from build123d import *

# Parameters (mm, degrees)
KES_EKSTR_ZYON1_DEPTH      = 49.846698967
KES_EKSTR_ZYON1_DEPTH_BACK = 49.846698967
PAH1_SIZE                  = 1


with BuildPart() as part:
    # Çizim1 → Döndür1 (revolve)
    with BuildSketch(Plane.XY, mode=Mode.PRIVATE) as d_nd_r1_sk:
        Polygon((0, 0), (0, 15), (-6, 15), (-6, 11), (-19, 11), (-19, 9), (-22, 9), (-22, 10), (-44, 10), (-44, 0), align=None)
    revolve(d_nd_r1_sk.sketch.rotate(Axis((0, 0, 0), (-1, 0, 0)), 90), axis=Axis((0, 0, 0), (-1, 0, 0)))

    # Çizim2 → Kes-Ekstrüzyon1 (cut, two sides: drawn at the far end of the back side and taken through both)
    with BuildSketch(Plane(origin=(0, 0, 0), x_dir=(1, 0, 0), z_dir=(0, 1, 0)).offset(-KES_EKSTR_ZYON1_DEPTH_BACK)):
        Polygon((0, 0), (0, 1), (-2, 1), (-2, -1), (0, -1), align=None)
    extrude(amount=KES_EKSTR_ZYON1_DEPTH + KES_EKSTR_ZYON1_DEPTH_BACK, mode=Mode.SUBTRACT)

    # Pah1
    pah1_edges = [part.edges().sort_by_distance(p)[0] for p in [
        (-44, 0, 10),
    ]]
    chamfer(pah1_edges, length=PAH1_SIZE)


solid = part.part
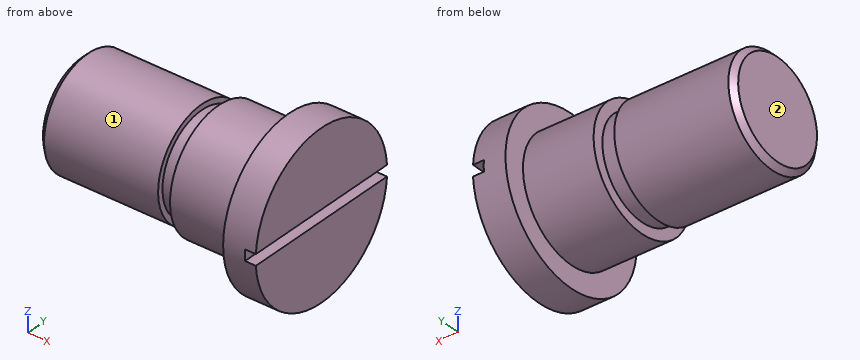
Can you work these out from the model? Positions are in its coordinate system, mm. Face numbers are marked on the shaded views. A direction names the side the tool comes from. Give positions to 0.01 mm unless a question says otherwise; leave off trailing zeros. Loops run counter-clockwise (first coordinate to the right, second up) from the corner with the lowest first, then second, coordinate; pieces in that order, holes last. Notation, with made-up numbers: M 34.5,77 L 91.5,77 A31 cw 91.5,111 Z; hole C 64,40.25 d3. An arc over 180 degrees is marked long. One line per item, written item: value. Start each with the question number.
1) If I drill on line 1 (Y direction, x = -38, z = 0.25); line 2 (X direction, y = -1.25, z = -11.25); line 3 (X direction, y = -3.5, z = -9.5), over which ranges is the centre line in solid material (lowest first)? Write a range as [from, to].
2) If we section it at D-D, the plane x = -5.5: Write out the boundary of the cut face in (y, z).
3) I'm going to push flat-ended pins straight in: pin 1 (12 mm diameter, centred on x = -11.5, z = -3, fed in from +Y); pin 2 (8 mm diameter, centred on x = -8, y = 10.5, fed in from +Z); pin 3 (1 mm diameter, centred on x = -7, z = -3, fed in from +Y). Where does each tip first touch, or does it pass through?
4) If we section it at B-B, the plane y = 0: Write out the boundary of the cut face in (x, z), and give its area (3 significant figures).
5) If we section it at C-C, the plane x = -16: Write out the boundary of the cut face in (y, z), and give its area (3 significant figures).
6) On a 3-axis mill with a long thin cutter (end or side, diameter ignored), from which of +Z, -Z, +X, -X, +Y, -Y can I reach the whole of each face in a straight line? I mean the marked faces 1 and 2. Say none if no direction works.
7) If we section it at A-A, the plane z = 0: Write out the boundary of the cut face in (x, y).
Completed:
1. line 1: y = [-10, 10]
1. line 2: x = [-6, 0]
1. line 3: x = [-19, 0]
2. outline: C 0,0 d30
3. pin 1: stops at y = 14.99
3. pin 2: stops at z = 13.25
3. pin 3: stops at y = 10.71
4. outline: M -44,-9 L -43,-10 L -22,-10 L -22,-9 L -19,-9 L -19,-11 L -6,-11 L -6,-15 L 0,-15 L 0,-1 L -2,-1 L -2,1 L 0,1 L 0,15 L -6,15 L -6,11 L -19,11 L -19,9 L -22,9 L -22,10 L -43,10 L -44,9 Z
4. area: 955 mm^2
5. outline: C 0,0 d22
5. area: 380 mm^2
6. face 1: -X
6. face 2: +Z, -Z, -X, +Y, -Y
7. outline: M -44,-9 L -43,-10 L -22,-10 L -22,-9 L -19,-9 L -19,-11 L -6,-11 L -6,-15 L -2,-15 L -2,15 L -6,15 L -6,11 L -19,11 L -19,9 L -22,9 L -22,10 L -43,10 L -44,9 Z
